from build123d import *

# Parameters (mm, degrees)
FILLET1_R           = 0.5
CHAMFER1_SIZE       = 0.5
CHAMFER2_SIZE       = 0.75
SKETCH4_R           = 1.5
CUT_EXTRUDE2_DEPTH  = 8.5
BOSS_EXTRUDE1_DEPTH = 8.5
CIRPATTERN1_COUNT   = 4


with BuildPart() as part:
    # Sketch1 → Revolve1 (revolve)
    with BuildSketch(Plane.XY):
        Polygon((0, 0), (2.5, 0), (2.5, 6.5), (2, 6.5), (2, 8.5), (2.5, 8.5), (2.5, 10), (2, 10), (2, 11.3), (4, 13.3), (4, 14.5), (2, 14.5), (2, 17.5), (0, 17.5), align=None)
    revolve(axis=Axis((0, -103.420301815, 0), (0, 1, 0)))

    # Fillet1
    fillet1_edges = [part.edges().sort_by_distance(p)[0] for p in [
        (-2, 8.5, 0),
    ]]
    fillet(fillet1_edges, radius=FILLET1_R - 0.0001)  # a hair under: the kernel refuses the full size

    # Chamfer1
    chamfer1_edges = [part.edges().sort_by_distance(p)[0] for p in [
        (-2.5, 0, 0),
    ]]
    chamfer(chamfer1_edges, length=CHAMFER1_SIZE)

    # Chamfer2
    chamfer2_edges = [part.edges().sort_by_distance(p)[0] for p in [
        (-2, 17.5, 0),
    ]]
    chamfer(chamfer2_edges, length=CHAMFER2_SIZE)

    # Sketch4 → Cut-Extrude2 (cut)
    with BuildSketch(Plane.XZ):
        Circle(SKETCH4_R)
    extrude(amount=-CUT_EXTRUDE2_DEPTH, mode=Mode.SUBTRACT)

    # Sketch6 → Boss-Extrude1 (add)
    with BuildSketch(Plane.XZ):
        with BuildLine():
            Line((-0.5, 1.414213562), (-0.5, 1.145643924))
            ThreePointArc((-0.5, 1.145643924), (0, 1.25), (0.5, 1.145643924))
            Line((0.5, 1.145643924), (0.5, 1.414213562))
            ThreePointArc((0.5, 1.414213562), (0, 1.5), (-0.5, 1.414213562))
        make_face()
    boss_extrude1 = extrude(amount=-BOSS_EXTRUDE1_DEPTH)

    # CirPattern1: Boss-Extrude1 ×4 about axis
    cirpattern1_axis = Axis((0, 0, 0), (0, 1, 0))
    for i in range(1, CIRPATTERN1_COUNT):
        add(boss_extrude1.rotate(cirpattern1_axis, i * 360 / CIRPATTERN1_COUNT))


solid = part.part
CAD build for the part. Positions are in the model's coordinates, mm. A direction names the side the tool comes from. Coordinates: 2 decimals unless noted, no trailing zeros. Order: outer loops, then holes, each group sorted by start corner. A loop starts at its lowest first (then second) coordinate and runs counter-clockwise, first axis right, second up.
Item 1: Drill centre lines: L1, parallel to Y at x = 1.75, z = 1.25; L2, parallel to X at y = 6, z = 0; L3, parallel to X at y = 4.25, z = -1. Where is each one in solid material? Low to high.
Check sheet entries:
L1: y = 0.15 to 6.5, 8.36 to 10, 11.45 to 14.5
L2: x = -2.5 to -1.25, 1.25 to 2.5
L3: x = -2.29 to -1.12, 1.12 to 2.29
Item 2: Two-plate mould, pull along Y, no slides. Class faces 1 (the face through (0, 11, 2)), 2 (the face through (0, 17.5, 0)), 3 (the face through (-0.01, 4.19, 1.25)): +Y half, -Y half, draft (parallel to the pull), parting line (faces both ways), or undercut.
Check sheet entries:
face 1: undercut
face 2: +Y half
face 3: draft
Item 3: Pin check, flat tips, straight feed: pin 1 Ø1.5 at (x, y) = (1, 10.5) entering from -Z; pin 2 Ø1.5 at (x, z) = (-2.5, -3) entering from +Y; pin 3 Ø4 at (y, z) = (8.5, 0.5) entering from +X. Stop position of each tip, or through.
Check sheet entries:
pin 1: stops at z = -2.46
pin 2: stops at y = 14.5
pin 3: stops at x = 2.5
Item 4: Band-saw the part on D-D on y = 14. List the corners of the cut face in (x, z).
Check sheet entries:
outline: circle Ø8 at (0, 0)
Item 5: 3-axis set-ups, long thin cutter, end or side, ignore diameter. For faces 4 (the face through (-0.54, 9.26, 2.44)), 5 (the face through (-2, 14.5, 1)), 6 (the face through (-0.867, 13.908, 3.905)), 7 (the face through (-1, 10, -2)): which of +Z, -Z, +X, -X, +Y, -Y reach the whole face in a straight line?
Check sheet entries:
face 4: -Y
face 5: +Y
face 6: +Y, -Y
face 7: none
Item 6: Band-saw the part on B-B on y = 1. List the corners of the cut face in (x, z), plus the area to 3 significant figures.
Check sheet entries:
outline: circle Ø5 at (0, 0); hole (-1.41, -0.5) arc R1.5 ccw to (-0.5, -1.41) - (-0.5, -1.15) arc R1.25 ccw to (0.5, -1.15) - (0.5, -1.41) arc R1.5 ccw to (1.41, -0.5) - (1.15, -0.5) arc R1.25 ccw to (1.15, 0.5) - (1.41, 0.5) arc R1.5 ccw to (0.5, 1.41) - (0.5, 1.15) arc R1.25 ccw to (-0.5, 1.15) - (-0.5, 1.41) arc R1.5 ccw to (-1.41, 0.5) - (-1.15, 0.5) arc R1.25 ccw to (-1.15, -0.5) - close
area: 13.6 mm2
